from build123d import *

# Parameters (mm, degrees)
CYLINDER026_R     = 1.2
CYLINDER026_DEPTH = 18.5
CYLINDER027_R     = 1.2
CYLINDER027_DEPTH = 18.5
BOX022_W          = 14
BOX022_H          = 8
BOX022_DEPTH      = 16.5


with BuildPart() as safetybuttonshookscrewcutter:
    # Cylinder026 → Cylinder026 (new body)
    with BuildSketch(Plane(origin=(-28.5, 0, 150.5), x_dir=(0, 0, -1), z_dir=(1, 0, 0))):
        Circle(CYLINDER026_R)
    extrude(amount=CYLINDER026_DEPTH)


with BuildPart() as obj1:
    # Cylinder027 → Cylinder027 (new body)
    with BuildSketch(Plane(origin=(-28.5, 0, 145.5), x_dir=(0, 0, -1), z_dir=(1, 0, 0))):
        Circle(CYLINDER027_R)
    extrude(amount=CYLINDER027_DEPTH)

    # Fusion013: union SafetyButtonsHookScrewCutter
    add(safetybuttonshookscrewcutter.part)


with BuildPart() as obj2:
    # Box022 → Box022 (new body)
    with BuildSketch(Plane(origin=(-28.5, -4, 137), x_dir=(1, 0, 0), z_dir=(0, 0, 1))):
        with Locations((7, 4)):
            Rectangle(BOX022_W, BOX022_H)
    extrude(amount=BOX022_DEPTH)

    # Cut051: cut obj1
    add(obj1.part, mode=Mode.SUBTRACT)


solid = obj2.part
Here's how the part is built. I have some questions about the finished solid (model axes, mm). Give positions to 0.01 mm unless a question says otherwise; leave off trailing zeros. Order: outer loops, then holes, each group sorted by start corner. A loop starts at its lowest first (then second) coordinate and runs counter-clockwise, first axis right, second up. Notation, with made-up numbers: (77, 0.25) -> (100, 0.25) arc R15 ccw to (100, 18.25) -> close; hole circle Ø4 at (-32, 79.5). An arc over 180 degrees is marked (long way). One line per item, written item: value. Start each with the question number.
1. Imagine slicing it at B-B, the plane y = 0. List the corners of the cut face in (x, z) for me.
2. Imagine slicing it at D-D, the plane z = 144.5. List the corners of the cut face in (x, y) for me, plus the area to 3 significant figures.
3. Imagine slicing it at A-A, the plane z = 150.5. List the corners of the cut face in (x, y) for me, plus the area to 3 significant figures.
4. Will this pin go through, and if not, where does the flat tip stop? pin 1 Ø1.9 at (y, z) = (0, 150.5) entering from -X (3 decimals).
5. Imagine slicing it at C-C, the plane x = -19.25. List the corners of the cut face in (y, z) for me.
6. I need wall thicknesses on probe 1 along Z at (x, y) = (-24, 0); probe 2 along Y at (x, z) = (-20.75, 150.5); probe 3 along Z at (x, y) = (-20.5, 1). Which ranges of each line are inside material? Lowest first, please. Write a range as from..to.
7. We'd pull the mould along Y, two halves only. Please class faces 1 (the face through (-21.6, 0.05, 151.7)), 2 (the face through (-22, 4, 145)), 3 (the face through (-28.5, 0, 143)), 4 (the face through (-22, -4, 145)): released by +Y, released by -Y, zero draft, split by the parting line, or undercut.
Values follow:
1. outline: (-28.5, 137) -> (-14.5, 137) -> (-14.5, 144.3) -> (-28.5, 144.3) -> close; (-28.5, 146.7) -> (-14.5, 146.7) -> (-14.5, 149.3) -> (-28.5, 149.3) -> close; (-28.5, 151.7) -> (-14.5, 151.7) -> (-14.5, 153.5) -> (-28.5, 153.5) -> close
2. outline: (-28.5, -4) -> (-14.5, -4) -> (-14.5, -0.66) -> (-28.5, -0.66) -> close; (-28.5, 0.66) -> (-14.5, 0.66) -> (-14.5, 4) -> (-28.5, 4) -> close
2. area: 93.4 mm2
3. outline: (-28.5, -4) -> (-14.5, -4) -> (-14.5, -1.2) -> (-28.5, -1.2) -> close; (-28.5, 1.2) -> (-14.5, 1.2) -> (-14.5, 4) -> (-28.5, 4) -> close
3. area: 78.4 mm2
4. pin 1: passes through
5. outline: (-4, 137) -> (4, 137) -> (4, 153.5) -> (-4, 153.5) -> close; hole circle Ø2.4 at (0, 145.5); hole circle Ø2.4 at (0, 150.5)
6. probe 1: z = 137..144.3, 146.7..149.3, 151.7..153.5
6. probe 2: y = -4..-1.2, 1.2..4
6. probe 3: z = 137..144.84, 146.16..149.84, 151.16..153.5
7. face 1: undercut
7. face 2: released by +Y
7. face 3: zero draft
7. face 4: released by -Y
